```python
from build123d import *

# Parameters (mm, degrees)
F0_R     = 26
F0_R_2   = 22
F1_DEPTH = 40


with BuildPart() as f1:
    # F0 (on Top) → F1 (new body)
    with BuildSketch(Plane.XY):
        Circle(F0_R)
        with BuildLine():
            ThreePointArc((-20.5, -3.5), (-20.646447, -3.853553), (-21, -4))
            Line((-21, -4), (-25, -4))
            ThreePointArc((-25, -4), (-25.353553, -3.853553), (-25.5, -3.5))
            Line((-25.5, -3.5), (-25.5, 3.5))
            ThreePointArc((-25.5, 3.5), (-25.353553, 3.853553), (-25, 4))
            Line((-25, 4), (-21, 4))
            ThreePointArc((-21, 4), (-20.646447, 3.853553), (-20.5, 3.5))
            Line((-20.5, 3.5), (-20.5, -3.5))
        make_face(mode=Mode.SUBTRACT)
        with Locations((2, 0)):
            Circle(F0_R_2, mode=Mode.SUBTRACT)
    extrude(amount=F1_DEPTH)


solid = f1.part
```
The listing builds one solid part. Answer for the finished solid, in the listing's coordinates (mm). A direction names the side the tool comes from. Coordinates: 2 decimals unless noted, no trailing zeros. Loops run counter-clockwise (first coordinate to the right, second up) from the corner with the lowest first, then second, coordinate; pieces in that order, holes last. Notation, with made-up numbers: (85.5, -27) -> (137.5, -27) arc R18 cw to (137.5, -10) -> close; hole circle Ø6 at (39.5, 0). An arc over 180 degrees is marked (long way). Return JSON: item names as keys, results as strings. Group by question number.
(1) Determine the mould class of faces 3 (the cylindrical face through (-20.633, -15.821, 19.72)), 4 (the flat face through (-23, -4, 20)), 5 (the flat face through (-19, 8, 0)) for opening direction Y: released by +Y, released by -Y, zero draft, split by the parting line, or undercut.
(2) A cutting plane is placed at A-A on y = 0. Write down the section's boundary in (x, z), and give its area (3 significant figures).
(3) Given pin 1 Ø6 at (y, z) = (8.5, 5.5) entering from +X; pin 2 Ø5 at (x, z) = (0.5, 9) entering from +Y; pin 3 Ø3 at (y, z) = (-18, 10.5) entering from -X, each flat-ended and moving along its own axis, determine where each tip first touches the part or whether it passes through.
(4) A cutting plane is placed at C-C on x = -18.5. Write down the section's boundary in (y, z), and give its area (3 significant figures).
(5) A cutting plane is placed at D-D on y = 8. Write down the section's boundary in (x, z).
(6) Which of the six approach directions +Z, -Z, +X, -X, +Y, -Y give full straight-line access (tool end or side, diameter ignored) to faces 1 (the flat face through (-23, 4, 20)), 2 (the flat face through (-19, 8, 40))?
(7) A cutting plane is placed at B-B on z = 3.5. Write down the section's boundary in (x, y), and give its area (3 significant figures).
(8) Find the intervals of material crossed by probe 1 along X at (y, z) = (-2, 9); probe 2 along X at (y, z) = (-1.5, 20.5); probe 3 along X at (y, z) = (-18.5, 10), in increasing order. Write a range as from..to.
The answers:
{
 "1": {"face 3": "split by the parting line", "face 4": "undercut", "face 5": "zero draft"},
 "2": {"outline": "(-26, 0) -> (-25.5, 0) -> (-25.5, 40) -> (-26, 40) -> close; (-20.5, 0) -> (-20, 0) -> (-20, 40) -> (-20.5, 40) -> close; (24, 0) -> (26, 0) -> (26, 40) -> (24, 40) -> close", "area": "120 mm^2"},
 "3": {"pin 1": "stops at x = 25.41", "pin 2": "stops at y = 26", "pin 3": "stops at x = -20.09"},
 "4": {"outline": "(-18.27, 0) -> (-7.98, 0) -> (-7.98, 40) -> (-18.27, 40) -> close; (7.98, 0) -> (18.27, 0) -> (18.27, 40) -> (7.98, 40) -> close", "area": "823 mm^2"},
 "5": {"outline": "(-24.74, 0) -> (-18.49, 0) -> (-18.49, 40) -> (-24.74, 40) -> close; (22.49, 0) -> (24.74, 0) -> (24.74, 40) -> (22.49, 40) -> close"},
 "6": {"face 1": "+Z, -Z", "face 2": "+Z, +X, -X, +Y, -Y"},
 "7": {"outline": "circle Ø52 at (0, 0); hole (-25.5, -3.5) arc R0.5 ccw to (-25, -4) -> (-21, -4) arc R0.5 ccw to (-20.5, -3.5) -> (-20.5, 3.5) arc R0.5 ccw to (-21, 4) -> (-25, 4) arc R0.5 ccw to (-25.5, 3.5) -> close; hole circle Ø44 at (2, 0)", "area": "563 mm^2"},
 "8": {"probe 1": "x = -25.92..-25.5, -20.5..-19.91, 23.91..25.92", "probe 2": "x = -25.96..-25.5, -20.5..-19.95, 23.95..25.96", "probe 3": "x = -18.27..-9.91, 13.91..18.27"}
}
